Input: part model. Units: mm. Frame: model coordinates. A direction names the side the tool comes from. Round coordinates to 2 decimals unless told otherwise and drop trailing zeros. Loops run counter-clockwise (first coordinate to the right, second up) from the corner with the lowest first, then second, coordinate; pieces in that order, holes last. Notation, with made-up numbers: M -33.75,52 L 10.25,52 A24 cw 10.25,73 Z; hole C -22,10.5 d8. An arc over 180 degrees is marked long. Put each result on its own line as item: value. Start each with the question number.
1) Section A-A on z = 50.5. State how many separate pieces and enclosed holes the cut face has, plus the area to 3 significant figures.
2) Section C-C on x = -45.5. Output: boundary loops of the cut face in (y, z), plus the area to 3 significant figures.
3) Reachability of faces 4 (the face through (-76, 75, 60)), 5 (the face through (-142, 2, 0)), 6 (the face through (30, -115, 20)) from +Z, -Z, +X, -X, +Y, -Y: full face, straight path, thin tool, end or side. Return the list, or none.
4) Draft query along Y for faces 1 (the face through (-3, 2, 80)), 2 (the face through (120, -75, 30)), 3 (the face through (-3, -125, 48)). Return one class per face: +Y half, -Y half, draft (parallel to the pull), parting line (faces both ways), or undercut.
5) Section D-D on y = 78. Output: boundary loops of the cut face in (x, z), plus the area to 3 significant figures.
6) Line query: probe 1 along X at (y, z) = (8, 16); probe 2 along X at (y, z) = (20, 57.5); probe 3 along Y at (x, z) = (47.5, 17.5). Output: solid intervals per line, ascending.
7) Pin query (flat end, axial travel): pin 1 (6 mm diameter, centred on x = 134, y = -44, fed in from -Z); pin 2 (18 mm diameter, centred on x = 62.5, y = -63, fed in from -Z). Return the tip coordinate at first contact, or that it passes through.
from build123d import *

# Parameters (mm, degrees)
F0_W     = 10
F0_H     = 115
F0_W_2   = 90
F0_H_2   = 20
F0_W_3   = 40
F0_H_3   = 60
F0_H_4   = 25
F0_W_4   = 30
F1_DEPTH = 80
F2_DEPTH = 60
F3_DEPTH = 40


with BuildPart() as f1:
    # F0 (on Top) → F1 (new body)
    with BuildSketch(Plane.XY):
        Polygon((-120, 125), (-250, 125), (-250, 115), (-240, 115), (-200, 115), (-120, 115), align=None)
        with Locations((-245, 57.5)):
            Rectangle(F0_W, F0_H)
        with Locations((-245, -57.5)):
            Rectangle(F0_W, F0_H)
        Polygon((-240, -115), (-250, -115), (-250, -125), (-120, -125), (-120, -115), (-200, -115), align=None)
        Polygon((-30, 125), (-120, 125), (-120, 115), (-120, 105), (-30, 105), align=None)
        Polygon((0, 125), (-30, 125), (-30, 105), (-30, 45), (-30, 25), (0, 25), align=None)
        with Locations((75, 115)):
            Rectangle(F0_W_2, F0_H_2)
        Polygon((30, 125), (0, 125), (0, 25), (30, 25), (30, 45), (30, 105), align=None)
        with Locations((-75, 35)):
            Rectangle(F0_W_2, F0_H_2)
        with Locations((-75, -35)):
            Rectangle(F0_W_2, F0_H_2)
        Polygon((-120, -115), (-120, -125), (-30, -125), (-30, -105), (-120, -105), align=None)
        Polygon((0, -125), (0, -25), (-30, -25), (-30, -45), (-30, -105), (-30, -125), align=None)
        Polygon((30, -25), (0, -25), (0, -125), (30, -125), (30, -105), (30, -45), align=None)
        with Locations((75, -35)):
            Rectangle(F0_W_2, F0_H_2)
        with Locations((75, 35)):
            Rectangle(F0_W_2, F0_H_2)
        with Locations((75, -115)):
            Rectangle(F0_W_2, F0_H_2)
        Polygon((250, 125), (120, 125), (120, 105), (120, 45), (120, 25), (120, 0), (250, 0), align=None)
        Polygon((250, -125), (250, 0), (120, 0), (120, -25), (120, -45), (120, -105), (120, -125), align=None)
        Polygon((-120, 105), (-120, 115), (-200, 115), (-200, 0), (-120, 0), (-120, 25), (-120, 45), align=None)
        Polygon((-120, 0), (-200, 0), (-200, -115), (-120, -115), (-120, -105), (-120, -45), (-120, -25), align=None)
        with Locations((-220, 57.5)):
            Rectangle(F0_W_3, F0_H)
        with Locations((-220, -57.5)):
            Rectangle(F0_W_3, F0_H)
        with Locations((-75, 75)):
            Rectangle(F0_W_2, F0_H_3)
        with Locations((-75, 12.5)):
            Rectangle(F0_W_2, F0_H_4)
        with Locations((-75, -12.5)):
            Rectangle(F0_W_2, F0_H_4)
        with Locations((-75, -75)):
            Rectangle(F0_W_2, F0_H_3)
        with Locations((-15, -12.5)):
            Rectangle(F0_W_4, F0_H_4)
        with Locations((-15, 12.5)):
            Rectangle(F0_W_4, F0_H_4)
        with Locations((15, 12.5)):
            Rectangle(F0_W_4, F0_H_4)
        with Locations((75, 12.5)):
            Rectangle(F0_W_2, F0_H_4)
        with Locations((75, -75)):
            Rectangle(F0_W_2, F0_H_3)
        with Locations((75, -12.5)):
            Rectangle(F0_W_2, F0_H_4)
        with Locations((15, -12.5)):
            Rectangle(F0_W_4, F0_H_4)
        with Locations((75, 75)):
            Rectangle(F0_W_2, F0_H_3)
    extrude(amount=F1_DEPTH)

    # F0 (on Top) → F2 (cut)
    with BuildSketch(Plane.XY):
        with Locations((-220, -57.5)):
            Rectangle(F0_W_3, F0_H)
        with Locations((-220, 57.5)):
            Rectangle(F0_W_3, F0_H)
        with Locations((75, -75)):
            Rectangle(F0_W_2, F0_H_3)
        with Locations((-75, -75)):
            Rectangle(F0_W_2, F0_H_3)
        with Locations((75, 75)):
            Rectangle(F0_W_2, F0_H_3)
        with Locations((-75, 75)):
            Rectangle(F0_W_2, F0_H_3)
        with Locations((-75, -12.5)):
            Rectangle(F0_W_2, F0_H_4)
        with Locations((-75, 12.5)):
            Rectangle(F0_W_2, F0_H_4)
        with Locations((75, -12.5)):
            Rectangle(F0_W_2, F0_H_4)
        with Locations((75, 12.5)):
            Rectangle(F0_W_2, F0_H_4)
    extrude(amount=F2_DEPTH, mode=Mode.SUBTRACT)

    # F0 (on Top) → F3 (cut)
    with BuildSketch(Plane.XY):
        Polygon((0, -125), (0, -25), (-30, -25), (-30, -45), (-30, -105), (-30, -125), align=None)
        Polygon((30, 125), (0, 125), (0, 25), (30, 25), (30, 45), (30, 105), align=None)
        Polygon((0, 125), (-30, 125), (-30, 105), (-30, 45), (-30, 25), (0, 25), align=None)
        with Locations((-15, 12.5)):
            Rectangle(F0_W_4, F0_H_4)
        with Locations((-15, -12.5)):
            Rectangle(F0_W_4, F0_H_4)
        with Locations((15, -12.5)):
            Rectangle(F0_W_4, F0_H_4)
        with Locations((15, 12.5)):
            Rectangle(F0_W_4, F0_H_4)
        Polygon((30, -25), (0, -25), (0, -125), (30, -125), (30, -105), (30, -45), align=None)
    extrude(amount=F3_DEPTH, mode=Mode.SUBTRACT)


solid = f1.part
Geometry results:
1. separate pieces: 1
1. enclosed holes: 7
1. area: 85,200 mm²
2. outline: M -125,0 L -105,0 L -105,60 L -45,60 L -45,0 L -25,0 L -25,60 L 25,60 L 25,0 L 45,0 L 45,60 L 105,60 L 105,0 L 125,0 L 125,80 L -125,80 Z
2. area: 9,800 mm²
3. face 4: -Z
3. face 5: -Z, +X, -X, +Y, -Y
3. face 6: -Z, +Y, -Y
4. face 1: draft
4. face 2: undercut
4. face 3: -Y half
5. outline: M -250,0 L -240,0 L -240,60 L -200,60 L -200,0 L -120,0 L -120,60 L -30,60 L -30,40 L 30,40 L 30,60 L 120,60 L 120,0 L 250,0 L 250,80 L -250,80 Z
5. area: 24,400 mm²
6. probe 1: x = -250 to -240, -200 to -120, 120 to 250
6. probe 2: x = -250 to -240, -200 to -120, -30 to 30, 120 to 250
6. probe 3: y = -125 to -105, -45 to -25, 25 to 45, 105 to 125
7. pin 1: stops at z = 0
7. pin 2: stops at z = 60
